Could you check a few things on this model? Use its own coordinates, in mm. Face numbers are marked on the shaded views. A direction names the side the tool comes from. Give positions to 0.01 mm unless a question says otherwise; leave off trailing zeros. Loops run counter-clockwise (first coordinate to the right, second up) from the corner with the lowest first, then second, coordinate; pieces in that order, holes last. Notation, with made-up numbers: (-14.5, -5.5) -> (43.5, -5.5) arc R9 ccw to (43.5, 10.5) -> close; hole circle Ø5 at (62, 74.5). An arc over 180 degrees is marked (long way). Write item = value, one per line. Start each with the question number.
1) On a 3-axis mill with a long thin cutter (end or side, diameter ignored), from which of +Z, -Z, +X, -X, +Y, -Y can I reach the whole of each face in a straight line? I mean the marked faces 1 and 2. Say none if no direction works.
2) I want a section at C-C (y = 0). Count the separate pieces of the cut face and the enclosed holes in it, and give its area (3 significant figures).
3) I need wall thicknesses on probe 1 along Y at (x, z) = (-11.65, -50.8); probe 2 along X at (y, z) = (1, 35.5); probe 3 along Y at (x, z) = (-4.5, -1.5). Which ranges of each line are inside material? Lowest first, please. Write a range as from..to.
4) I want a section at B-B (z = 0). List the corners of the cut face in (x, y) for me.
5) I want a section at A-A (x = 7). List the corners of the cut face in (y, z) for me, and give its area (3 significant figures).
6) I'm going to push a flat-ended pin straight in: pin 1 Ø4.5 at (y, z) = (15.88, -27.5) entering from -X. Where does the tip first touch, or does it pass through?
7) If we mould it in two halves opening along Y, with no side actions, what happens to the marked faces 3, 4, 5 and 6? For each: +Y half, -Y half, draft (parallel to the pull), parting line (faces both ways), or undercut.
Autodesk Inventor part; units mm, degrees
ref_plane "YZ Plane" through (0, 0, 0) normal (1, 0, 0) x (0, 1, 0)
ref_plane "XZ Plane" through (0, 0, 0) normal (0, 1, 0) x (-1, 0, 0)
ref_plane "XY Plane" through (0, 0, 0) normal (0, 0, 1) x (1, 0, 0)
sketch "Sketch1" plane through (0, 0, 0) normal (0, 0, 1) x (1, 0, 0)
  line L0 (-12.7, -25.4) -> (12.7, -25.4)
  line L1 (12.7, -25.4) -> (12.7, 25.4)
  line L2 (12.7, 25.4) -> (-12.7, 25.4)
  line L3 (-12.7, 25.4) -> (-12.7, -25.4)
  line L4 (-12.7, -25.4) -> (12.7, 25.4) construction
  line L5 (12.7, -25.4) -> (-12.7, 25.4) construction
  line L6 (-11.1125, 23.8125) -> (11.1125, 23.8125)
  line L7 (11.1125, 23.8125) -> (11.1125, -23.8125)
  line L8 (11.1125, -23.8125) -> (-11.1125, -23.8125)
  line L9 (-11.1125, -23.8125) -> (-11.1125, 23.8125)
  point P0 (0, 0)
  dimension "width" = 25.4
  dimension "height" = 50.8
  dimension "thickness" = 1.5875
extrude "Extrusion1" add sketch "Sketch1" along normal mid plane 127
sketch "Sketch2" plane through (-12.7, -25.4, 63.5) normal (-1, 0, 0) x (0, 0, 1)
  circle A0 centre (-63.5, 25.4) radius 31.75 construction
  line L0 (-127, 0) -> (-127, 50.8)
  line L1 (-63.5, 50.8) -> (-63.5, 0) construction
  line L2 (0, 0) -> (-127, 0) construction
  line L3 (-127, 50.8) -> (0, 50.8) construction
  point P0 (-63.5, 57.15)
  point P1 (-90.9963, 41.275)
  point P2 (-90.9963, 9.525)
  point P3 (-63.5, -6.35)
  point P4 (-36.0037, 9.525)
  point P5 (-36.0037, 41.275)
  point P6 (-114.3, 38.1)
  point P7 (-114.3, 25.4)
  point P8 (-114.3, 12.7)
  point P9 (-12.7, 38.1)
  point P10 (-12.7, 25.4)
  point P11 (-12.7, 12.7)
  dimension "d5" = 63.5
  dimension "d8" = 360
  dimension "d17" = 12.7
  dimension "d18" = 12.7
  dimension "d19" = 12.7
hole "Hole1" at (-12.7, 15.875, -27.4963) at (-12.7, -15.875, -27.4963) at (-12.7, -15.875, 27.4963) at (-12.7, 15.875, 27.4963) at (-12.7, 12.7, -50.8) at (-12.7, 0, -50.8) at (-12.7, -12.7, -50.8) at (-12.7, -12.7, 50.8) at (-12.7, 0, 50.8) at (-12.7, 12.7, 50.8) direction (1, 0, 0) diameter 5.1054 end through all
sketch "Sketch3" plane through (12.7, -25.4, 63.5) normal (1, 0, 0) x (0, 0, -1)
  circle A0 centre (63.5, 25.4) radius 19.05
  dimension "d20" = 38.1
extrude "Extrusion2" cut sketch "Sketch3" against normal through all
properties part number "GP4-002" material "Aluminum 6061"
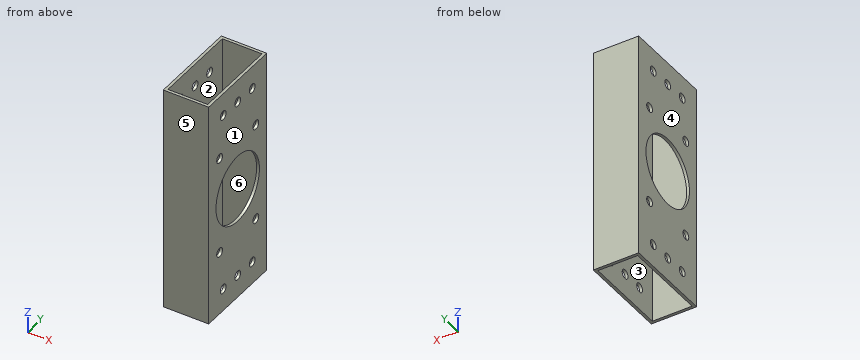
Answer list:
q1.face_1 = +Z, -Z, +X, +Y, -Y
q1.face_2 = +Z, -Z
q2.separate_pieces = 8
q2.enclosed_holes = 0
q2.area = 250 mm^2
q3.probe_1 = -25.4..-15.25, -10.15..-2.55, 2.55..10.15, 15.25..25.4
q3.probe_2 = -12.7..-11.11, 11.11..12.7
q3.probe_3 = -25.4..-23.81, 23.81..25.4
q4.outline = (-12.7, -25.4) -> (12.7, -25.4) -> (12.7, -19.05) -> (11.11, -19.05) -> (11.11, -23.81) -> (-11.11, -23.81) -> (-11.11, -19.05) -> (-12.7, -19.05) -> close; (-12.7, 19.05) -> (-11.11, 19.05) -> (-11.11, 23.81) -> (11.11, 23.81) -> (11.11, 19.05) -> (12.7, 19.05) -> (12.7, 25.4) -> (-12.7, 25.4) -> close
q5.outline = (-25.4, -63.5) -> (-23.81, -63.5) -> (-23.81, 63.5) -> (-25.4, 63.5) -> close; (23.81, -63.5) -> (25.4, -63.5) -> (25.4, 63.5) -> (23.81, 63.5) -> close
q5.area = 403 mm^2
q6.pin_1 = through
q7.face_3 = undercut
q7.face_4 = draft
q7.face_5 = -Y half
q7.face_6 = undercut
